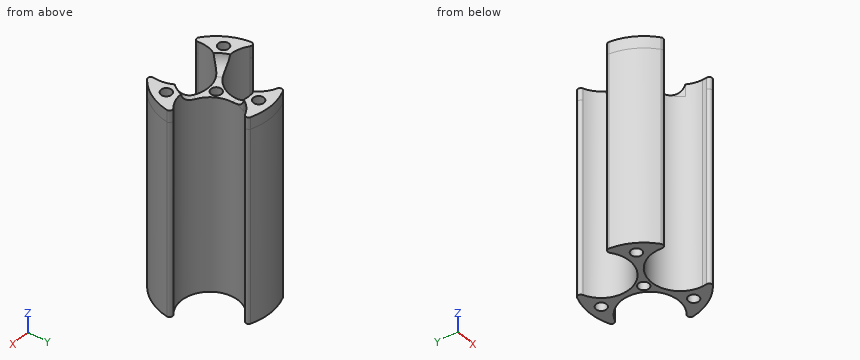
```python
from build123d import *

# Parameters (mm, degrees)
SKETCH_1_R      = 1.75
EXTRUDE_1_DEPTH = 65
FILLET_1_R      = 1
SKETCH_2_R      = 1.75
EXTRUDE_2_DEPTH = 4
FILLET_2_R      = 5


with BuildPart() as part:
    # Эскиз1 → Бобышка-Вытянуть1 (new body)
    with BuildSketch(Plane.XY):
        with BuildLine():
            ThreePointArc((8.733013025, -15.739583333), (15.511193288, -9.132517877), (18, 0))
            ThreePointArc((18, 0), (17.999346369, 0.153395838), (17.997385524, 0.306780536))
            ThreePointArc((17.997385524, 0.306780536), (2.165063509, 1.25), (9.264372499, 15.432802798))
            ThreePointArc((9.264372499, 15.432802798), (0, 18), (-9.264372499, 15.432802798))
            ThreePointArc((-9.264372499, 15.432802798), (-3.287188474, 12.30613363), (-0.892304845, 6))
            ThreePointArc((-0.892304845, 6), (-7.392160386, -3.013830108), (-17.997385524, 0.306780536))
            ThreePointArc((-17.997385524, 0.306780536), (-15.588457268, -9), (-8.733013025, -15.739583333))
            ThreePointArc((-8.733013025, -15.739583333), (-1.908713738, -2.693721911), (9.5, -12))
            ThreePointArc((9.5, -12), (9.306278089, -13.908713738), (8.733013025, -15.739583333))
        make_face()
        with Locations((-12.124355653, -7)):
            Circle(SKETCH_1_R, mode=Mode.SUBTRACT)
        with Locations((12.124355653, -7)):
            Circle(SKETCH_1_R, mode=Mode.SUBTRACT)
        Circle(SKETCH_1_R, mode=Mode.SUBTRACT)
        with Locations((0, 14)):
            Circle(SKETCH_1_R, mode=Mode.SUBTRACT)
    extrude(amount=EXTRUDE_1_DEPTH)

    # Скругление1
    fillet_1_edges = [part.edges().sort_by_distance(p)[0] for p in [
        (17.997385524, 0.306780536, 32.5),
        (8.733013025, -15.739583333, 32.5),
        (-8.733013025, -15.739583333, 32.5),
        (-17.997385524, 0.306780536, 32.5),
        (-9.264372499, 15.432802798, 32.5),
        (9.264372499, 15.432802798, 32.5),
    ]]
    fillet(fillet_1_edges, radius=FILLET_1_R)

    # Эскиз2 → Бобышка-Вытянуть2 (add)
    # profile 1 of 3: a face of its own
    with BuildSketch(Plane.XY.offset(65)):
        with BuildLine():
            ThreePointArc((6.822193962, 14.803653121), (7.446391133, 15.728518462), (6.825592394, 16.655668359))
            ThreePointArc((6.825592394, 16.655668359), (0, 18), (-6.825592394, 16.655668359))
            ThreePointArc((-6.825592394, 16.655668359), (-7.446391133, 15.728518462), (-6.822193962, 14.803653121))
            ThreePointArc((-6.822193962, 14.803653121), (-4.168730882, 13.177543251), (-2.183145185, 10.781181619))
            ThreePointArc((-2.183145185, 10.781181619), (0, 11), (2.183145185, 10.781181619))
            ThreePointArc((2.183145185, 10.781181619), (4.168730882, 13.177543251), (6.822193962, 14.803653121))
        make_face()
        with Locations((0, 14)):
            Circle(SKETCH_2_R, mode=Mode.SUBTRACT)
    # profile 2 of 3: a face of its own
    with BuildSketch(Plane.XY.offset(65)):
        with BuildLine():
            ThreePointArc((17.837028113, -2.41669777), (17.344492118, -1.415495343), (16.231436653, -1.49363328))
            ThreePointArc((16.231436653, -1.49363328), (13.496452656, -2.97854478), (10.428349757, -3.499931619))
            ThreePointArc((10.428349757, -3.499931619), (9.526279442, -5.5), (8.245204572, -7.28125))
            ThreePointArc((8.245204572, -7.28125), (9.1809434, -9.558631883), (9.5, -12))
            ThreePointArc((9.5, -12), (9.477283513, -12.656579941), (9.409242691, -13.310019841))
            ThreePointArc((9.409242691, -13.310019841), (9.898100985, -14.313023118), (11.011435719, -14.238970588))
            ThreePointArc((11.011435719, -14.238970588), (15.588457268, -9), (17.837028113, -2.41669777))
        make_face()
        with Locations((12.124355653, -7)):
            Circle(SKETCH_2_R, mode=Mode.SUBTRACT)
    # profile 3 of 3: a face of its own
    with BuildSketch(Plane.XY.offset(65)):
        with BuildLine():
            ThreePointArc((-10.428349757, -3.499931619), (-13.496452656, -2.97854478), (-16.231436653, -1.49363328))
            ThreePointArc((-16.231436653, -1.49363328), (-17.344492118, -1.415495343), (-17.837028113, -2.41669777))
            ThreePointArc((-17.837028113, -2.41669777), (-15.588457268, -9), (-11.011435719, -14.238970588))
            ThreePointArc((-11.011435719, -14.238970588), (-9.898100985, -14.313023118), (-9.409242691, -13.310019841))
            ThreePointArc((-9.409242691, -13.310019841), (-9.327721774, -10.198998471), (-8.245204572, -7.28125))
            ThreePointArc((-8.245204572, -7.28125), (-9.526279442, -5.5), (-10.428349757, -3.499931619))
        make_face()
        with Locations((-12.124355653, -7)):
            Circle(SKETCH_2_R, mode=Mode.SUBTRACT)
    extrude(amount=EXTRUDE_2_DEPTH)

    # Скругление2
    # the kernel refuses this fillet: 5 mm, written as the material it adds along each edge
    with BuildSketch(Plane(origin=(0, 0, 65), x_dir=(0.26290330045081145, -0.9648221880803066, 0), z_dir=(0.9648221880803066, 0.26290330045081145, 0))) as fillet_2_piece_1_section:
        with BuildLine():
            CenterArc((6.101020514, -5), FILLET_2_R, 11.536959033, 78.463040967)
            Line((6.101020514, 0), (6.101020514, 0.1))
            Line((6.101020514, 0.1), (11, 0.1))
            Line((11, 0.1), (11.1, 0))
            ThreePointArc((11.1, 0), (11.1, -2), (11.09797959, -3.98))
            Line((11.09797959, -3.98), (11, -4))
        make_face()
    fillet_2_piece_1 = revolve(axis=Axis((0, 0, 65), (0, 0, -1)), revolution_arc=150.484807428, mode=Mode.PRIVATE)
    fillet_2_piece_1 = fillet_2_piece_1 - Plane(origin=(-10.392304845, 6, 66.122013519), x_dir=(0.1187297206541081, 0.9929266102957446, 0), z_dir=(0, 0, -1)) * Cylinder(9.5, 45, mode=Mode.PRIVATE)
    fillet_2_piece_1 = fillet_2_piece_1 - Plane(origin=(0, -12, 66.122013519), x_dir=(-0.9192645289367253, -0.3936403508772196, 0), z_dir=(0, 0, -1)) * Cylinder(9.5, 45, mode=Mode.PRIVATE)
    add(fillet_2_piece_1)
    with BuildSketch(Plane(origin=(0, 0, 65), x_dir=(0.7041088747870229, 0.7100920309693333, 0), z_dir=(-0.7100920309693333, 0.7041088747870229, 0))) as fillet_2_piece_2_section:
        with BuildLine():
            CenterArc((6.101020514, -5), FILLET_2_R, 11.536959033, 78.463040967)
            Line((11, -4), (11.09797959, -3.98))
            ThreePointArc((11.09797959, -3.98), (11.1, -2), (11.1, 0))
            Line((11.1, 0), (11, 0.1))
            Line((11, 0.1), (6.101020514, 0.1))
            Line((6.101020514, 0.1), (6.101020514, 0))
        make_face()
    fillet_2_piece_2 = revolve(axis=Axis((0, 0, 65), (0, 0, -1)), revolution_arc=150.484807428, mode=Mode.PRIVATE)
    fillet_2_piece_2 = fillet_2_piece_2 - Plane(origin=(10.392304845, 6, 66.122013516), x_dir=(0.8005348082826462, -0.5992862594185411, 0), z_dir=(0, 0, -1)) * Cylinder(9.5, 45, mode=Mode.PRIVATE)
    fillet_2_piece_2 = fillet_2_piece_2 - Plane(origin=(0, -12, 66.122013516), x_dir=(-0.9192645289367253, -0.3936403508772196, 0), z_dir=(0, 0, -1)) * Cylinder(9.5, 45, mode=Mode.PRIVATE)
    add(fillet_2_piece_2)
    with BuildSketch(Plane(origin=(0, 0, 65), x_dir=(-0.9670121752378409, 0.2547301571109701, 0), z_dir=(-0.2547301571109701, -0.9670121752378409, 0))) as fillet_2_piece_3_section:
        with BuildLine():
            CenterArc((6.101020514, -5), FILLET_2_R, 11.536959033, 78.463040967)
            Line((6.101020514, 0), (6.101020514, 0.1))
            Line((6.101020514, 0.1), (11, 0.1))
            Line((11, 0.1), (11.1, 0))
            ThreePointArc((11.1, 0), (11.1, -2), (11.09797959, -3.98))
            Line((11.09797959, -3.98), (11, -4))
        make_face()
    fillet_2_piece_3 = revolve(axis=Axis((0, 0, 65), (0, 0, -1)), revolution_arc=150.484807428, mode=Mode.PRIVATE)
    fillet_2_piece_3 = fillet_2_piece_3 - Plane(origin=(10.392304845, 6, 66.122013519), x_dir=(0.8005348082826462, -0.5992862594185411, 0), z_dir=(0, 0, -1)) * Cylinder(9.5, 45, mode=Mode.PRIVATE)
    fillet_2_piece_3 = fillet_2_piece_3 - Plane(origin=(-10.392304845, 6, 66.122013519), x_dir=(0.1187297206541081, 0.9929266102957446, 0), z_dir=(0, 0, -1)) * Cylinder(9.5, 45, mode=Mode.PRIVATE)
    add(fillet_2_piece_3)


solid = part.part
```
The listing builds one solid part. Answer for the finished solid, in the listing's coordinates (mm). Give positions to 0.01 mm unless a question says otherwise; leave off trailing zeros. Write each loop counter-clockwise with the first axis right and the second up, starting at its lowest first coordinate (ties: lowest second). Pieces come first, ordered by that corner, then holes. Notation, with made-up numbers: (19, 83.25) -> (66, 83.25) arc R30 ccw to (66, 115.25) -> close; hole circle Ø4 at (-14, -31.75). An arc over 180 degrees is marked (long way). Use one line per item in the form item = value.
1) Section C-C on y = 14 is taken. Write down the section's boundary in (x, z).
Result:
outline = (-5.27, 0) -> (-1.75, 0) -> (-1.75, 69) -> (-5.27, 69) -> close; (1.75, 0) -> (5.27, 0) -> (5.27, 69) -> (1.75, 69) -> close
2) Each of these flat-tipped pins is pushed along its axis until it touches: P1, Ø3, axis at x = -12.12, y = -7, coming from the -Z side; P2, Ø1, axis at x = -11, z = 37, coming from the +Y side; P3, Ø8, axis at x = -10, z = 48.5, coming from the +Y side; P4, Ø5, axis at x = 0, y = 1, coming from the +Z side. Where does it stop, or does it pass through?
Result:
P1 = through
P2 = -3.44
P3 = 16.97
P4 = 65
3) Section A-A on y = 0 is taken. Write down the section's boundary in (x, z), plus the area to 3 significant figures.
Result:
outline = (-3.03, 0) -> (-1.75, 0) -> (-1.75, 65) -> (-3.03, 65) -> close; (1.75, 0) -> (3.03, 0) -> (3.03, 65) -> (1.75, 65) -> close
area = 166 mm²
4) Straight lines are drawn through the part: probe 1 along Y at (x, z) = (0.5, 11); probe 2 along X at (y, z) = (-6, 61); probe 3 along Y at (x, z) = (-12, 64.5). For each, find the intervals that lie inside material, in ascending order.
Result:
probe_1 = -2.51 to -1.68, 1.68 to 12.32, 15.68 to 17.99
probe_2 = -16.97 to -13.56, -10.69 to -7.37, 7.37 to 10.69, 13.56 to 16.97
probe_3 = -13.42 to -8.75, -5.25 to -3.36
5) Section B-B on x = 13 is taken. Write down the section's boundary in (y, z).
Result:
outline = (-12.45, 0) -> (-8.52, 0) -> (-8.52, 69) -> (-12.45, 69) -> close; (-5.48, 0) -> (-3.14, 0) -> (-3.14, 69) -> (-5.48, 69) -> close
